Design review of the part built by this model. Coordinates are the model's own, in mm. A direction names the side the tool comes from. Coordinates: 2 decimals unless noted, no trailing zeros. Loops run counter-clockwise (first coordinate to the right, second up) from the corner with the lowest first, then second, coordinate; pieces in that order, holes last. Notation, with made-up numbers: (22, 84.25) - (60, 84.25) arc R23 ccw to (60, 116.25) - close; hole circle Ø6 at (-19, 0.25). An arc over 180 degrees is marked (long way). Answer in a Markdown table with one row per item. Add a question column.
(1) We need section B-B, the plane x = -11.5. Write out the cut boundary in (y, z), plus the area to 3 significant figures.
(2) For faces 1 (the face through (-18.3, -8.85, 1.46)), 2 (the face through (-23.29, 11.55, 0.18)), 3 (the face through (26.4, -11.9, 9.2)), 4 (the face through (4, 0, 3)), list the 3-axis set-ups (+Z, -Z, +X, -X, +Y, -Y) from which the entire face can be reached by the end or side of a thin tool; tool diameter is ignored.
(3) The part is to be moulded in two halves that separate along Y. For faces 5 (the face through (-0.1, 15, 2.6)), 6 (the face through (-20.79, 12.77, 0.91)), 7 (the face through (0, 4, 0)), say which applies: released by +Y, released by -Y, zero draft, split by the parting line, or undercut.
(4) Clearance check with flat-ended pins moving along their axes: pin 1 (1.1 mm diameter, centred on x = -20, y = 5, fed in from +Z); pin 2 (6.5 mm diameter, centred on y = -1, z = 7.5, fed in from -X) (3 decimals). State where each tip first meets the part, or that it passes through.
(5) We need section A-A, the plane z = 8. Write out the cut boundary in (x, y) (3 decimals).
(6) To check wall thickness, follow L1, parallel to Y at x = 26, z = 8; L2, parallel to Y at x = 0, z = 1.5; L3, parallel to Z at x = 12, y = -10. State the ranges of each line that lie inside material, in increasing order. Write a range as [from, to].
from build123d import *

# Parameters (mm, degrees)
SKETCH1_W           = 55.85
SKETCH1_H           = 30
BOSS_EXTRUDE1_DEPTH = 3
SKETCH2_W           = 8.4
SKETCH2_H           = 30
BOSS_EXTRUDE2_DEPTH = 3
CHAMFER1_SIZE       = 5
CHAMFER1_SIZE2      = 7
SKETCH3_R           = 1.5
CUT_EXTRUDE1_DEPTH  = 3
CHAMFER2_SIZE       = 3
CUT_EXTRUDE2_START  = -3
CUT_EXTRUDE2_DEPTH  = 8
SKETCH5_W           = 3
SKETCH5_H           = 30
BOSS_EXTRUDE3_DEPTH = 8
SKETCH6_R           = 1.5
CUT_EXTRUDE3_DEPTH  = 8
SKETCH7_R           = 1.5
CUT_EXTRUDE4_DEPTH  = 34.553027062


with BuildPart() as part:
    # Sketch1 → Boss-Extrude1 (new body)
    with BuildSketch(Plane.XY):
        Rectangle(SKETCH1_W, SKETCH1_H)
    extrude(amount=BOSS_EXTRUDE1_DEPTH)

    # Sketch2 → Boss-Extrude2 (add)
    with BuildSketch(Plane.XY.offset(3)):
        with Locations((-23.725, 0)):
            Rectangle(SKETCH2_W, SKETCH2_H)
    extrude(amount=BOSS_EXTRUDE2_DEPTH)

    # Chamfer1
    chamfer1_edges = [part.edges().sort_by_distance(p)[0] for p in [
        (-27.925, 0, 6),
    ]]
    chamfer1_side = [part.faces().sort_by_distance(p)[0] for p in [
        (-27.925, 0, 3),
    ]]
    chamfer(chamfer1_edges, length=CHAMFER1_SIZE, length2=CHAMFER1_SIZE2, reference=chamfer1_side[0])

    # Sketch3 → Cut-Extrude1 (cut)
    with BuildSketch(Plane(origin=(-9.907094595, 0, 13.869932432), x_dir=(0.8137334712067354, 0, 0.5812381937190957), z_dir=(-0.5812381937190957, 0, 0.8137334712067354))):
        with Locations((-16.539943723, 10)):
            Circle(SKETCH3_R)
        with Locations((-16.539943723, -10)):
            Circle(SKETCH3_R)
    extrude(amount=-CUT_EXTRUDE1_DEPTH, mode=Mode.SUBTRACT)

    # Chamfer2
    chamfer2_edges = [part.edges().sort_by_distance(p)[0] for p in [
        (-19.525, 0, 3),
    ]]
    chamfer(chamfer2_edges, length=CHAMFER2_SIZE - 0.0001)  # a hair under: the kernel refuses the full size

    # Sketch4 → Cut-Extrude2 (cut)
    with BuildSketch(Plane(origin=(-9.907094595, 0, 13.869932432), x_dir=(0.8137334712067354, 0, 0.5812381937190959), z_dir=(-0.5812381937190958, 0, 0.8137334712067353)).offset(CUT_EXTRUDE2_START)):
        Polygon((-14.730494791, 7.39055027), (-13.3753695, 10.262303877), (-15.184818432, 12.871753607), (-18.349392655, 12.60944973), (-19.704517945, 9.737696123), (-17.895069013, 7.128246393), align=None)
        Polygon((-14.730494791, -7.39055027), (-17.895069013, -7.128246393), (-19.704517945, -9.737696123), (-18.349392655, -12.60944973), (-15.184818432, -12.871753607), (-13.3753695, -10.262303877), align=None)
    extrude(amount=-CUT_EXTRUDE2_DEPTH, mode=Mode.SUBTRACT)

    # Sketch5 → Boss-Extrude3 (add)
    with BuildSketch(Plane.XY.offset(3)):
        with Locations((26.425, 0)):
            Rectangle(SKETCH5_W, SKETCH5_H)
    extrude(amount=BOSS_EXTRUDE3_DEPTH)

    # Sketch6 → Cut-Extrude3 (cut)
    with BuildSketch(Plane(origin=(27.925, 0, 0), x_dir=(0, 0, -1), z_dir=(1, 0, 0))):
        with Locations((-8, 11)):
            Circle(SKETCH6_R)
        with Locations((-8, -11)):
            Circle(SKETCH6_R)
    extrude(amount=-CUT_EXTRUDE3_DEPTH, mode=Mode.SUBTRACT)

    # Sketch7 → Cut-Extrude4 (cut, through all)
    with BuildSketch(Plane(origin=(0, 0, 0), x_dir=(-1, 0, 0), z_dir=(0, 0, -1))):
        Circle(SKETCH7_R)
    extrude(amount=-CUT_EXTRUDE4_DEPTH, mode=Mode.SUBTRACT)


solid = part.part
Responses:
| question | item | result |
|---|---|---|
| 1 | outline | (-15, 0) - (15, 0) - (15, 3) - (-15, 3) - close |
| 1 | area | 90.0 mm2 |
| 2 | face 1 | -Z |
| 2 | face 2 | none |
| 2 | face 3 | +X, -X |
| 2 | face 4 | +Z, +Y, -Y |
| 3 | face 5 | released by +Y |
| 3 | face 6 | undercut |
| 3 | face 7 | zero draft |
| 4 | pin 1 | stops at z = 6 |
| 4 | pin 2 | stops at x = -23.375 |
| 5 | outline | (24.925, -15) - (27.925, -15) - (27.925, -12.5) - (24.925, -12.5) - close; (24.925, -9.5) - (27.925, -9.5) - (27.925, 9.5) - (24.925, 9.5) - close; (24.925, 12.5) - (27.925, 12.5) - (27.925, 15) - (24.925, 15) - close |
| 6 | L1 | y = [-15, -12.5], [-9.5, 9.5], [12.5, 15] |
| 6 | L2 | y = [-15, -1.5], [1.5, 15] |
| 6 | L3 | z = [0, 3] |
